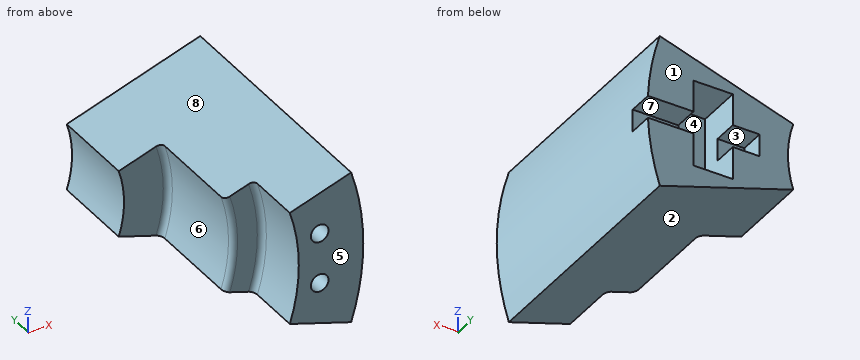
Autodesk Inventor part; units mm, degrees
ref_plane "YZ Plane" through (0, 0, 0) normal (1, 0, 0) x (0, 1, 0)
ref_plane "XZ Plane" through (0, 0, 0) normal (0, 1, 0) x (-1, 0, 0)
ref_plane "XY Plane" through (0, 0, 0) normal (0, 0, 1) x (1, 0, 0)
sketch "Эскиз3" plane through (0, 0, 0) normal (0, 0, 1) x (1, 0, 0)
  line L0 (28.4814, 0) -> (32, 0)
  line L1 (26.4814, 18.1962) -> (19.4814, 18.1962)
  line L2 (19.4814, 18.1962) -> (19.4814, 33.1962)
  line L3 (27.4814, 17.1962) -> (27.4814, 1)
  line L4 (33, -1) -> (33, -10.35)
  line L5 (33, -10.35) -> (44.4955, -10.35)
  line L6 (109.4355, -10.35) -> (-108.0344, -10.35)
  arc A0 (33, -1) -> (32, 0) centre (32, -1) ccw
  arc A1 (27.4814, 1) -> (28.4814, 0) centre (28.4814, 1) ccw
  arc A2 (27.4814, 17.1962) -> (26.4814, 18.1962) centre (26.4814, 17.1962) ccw
  line L7 (19.4814, 33.1962) -> (44.4955, 33.1962)
  line L8 (44.4955, 33.1962) -> (44.4955, -10.35)
  point P0 (27.4814, 18.1962)
  point P1 (27.4814, 0)
  dimension "d25" = 8
  dimension "d42" = 15
  dimension "d44" = 1
  dimension "d45" = 1
  dimension "d54" = 3.5186
  dimension "d55" = 25.0142
sketch "Эскиз4" plane through (0, 0, 0) normal (0, 1, 0) x (-1, 0, 0)
  arc A0 (-24.7386, 8) -> (-24.7386, -8) centre (0, 0) ccw
  dimension "d31" = 26
sweep "Сдвиг1" add profiles "Эскиз3" path "Эскиз4"
sketch "Эскиз8" plane through (0, -10.35, 0) normal (0, -1, 0) x (1, 0, 0)
  arc A0 (31.399, -10.1538) -> (31.399, 10.1538) centre (0, 0) ccw
  arc A1 (35.205, -11.3846) -> (35.205, 11.3846) centre (0, 0) ccw construction
  line L0 (42.3369, -13.6909) -> (31.399, -10.1538)
  circle A2 centre (36.723, -4.5186) radius 1.575
  circle A3 centre (36.723, 4.5186) radius 1.575
  line L1 (31.399, 10.1538) -> (42.3369, 13.6909)
  point P0 (0, 0)
  dimension "d46" = 4
  dimension "d47" = 3.15
  dimension "d48" = 3.15
  dimension "d49" = 7
  dimension "d50" = 7
extrude "Выдавливание4" cut sketch "Эскиз8" against normal blind 10
sketch "Эскиз9" plane through (0, 33.1962, 0) normal (0, 1, 0) x (1, 0, 0)
  point P0 (0, 0)
ref_plane "РабПлоскость1" through (0, -10.35, 0) normal (0, 0, 1) x (0, 1, 0)
sketch "Эскиз10" plane through (0, -10.35, 0) normal (0, 0, 1) x (0, 1, 0)
  line L0 (47.9462, -48.5362) -> (39.1462, -48.5362)
  line L1 (39.1462, -48.5362) -> (39.1462, -24.5362)
  line L2 (39.1462, -24.5362) -> (47.9462, -24.5362)
  line L3 (47.9462, -24.5362) -> (47.9462, -48.5362)
  line L4 (43.5462, -42.3369) -> (43.5462, -18.5362)
  line L5 (47.9462, -48.5362) -> (39.1462, -24.5362) construction
  line L6 (39.1462, -48.5362) -> (47.9462, -24.5362) construction
  line L7 (28.5462, -18.5362) -> (43.5462, -18.5362)
  point P0 (10.35, 0)
  point P1 (43.5462, -36.5362)
  dimension "d61" = 8.8
  dimension "d68" = 24
  dimension "d69" = 6
extrude "Выдавливание5" cut sketch "Эскиз10" along normal mid plane 4
sketch "Эскиз11" plane through (0, 33.1962, 0) normal (0, 1, 0) x (1, 0, 0)
  line L0 (34.8211, -6.1599) -> (30.8211, -6.1599)
  line L1 (30.8211, -6.1599) -> (30.8211, -0.8676)
  line L2 (30.8211, -0.8676) -> (34.8211, -0.8676)
  line L3 (34.8211, -0.8676) -> (34.8211, -6.1599)
  line L4 (30.8211, 6.3599) -> (34.8211, 6.3599)
  line L5 (34.8211, 6.3599) -> (34.8211, 1.0676)
  line L6 (34.8211, 1.0676) -> (30.8211, 1.0676)
  line L7 (30.8211, 1.0676) -> (30.8211, 6.3599)
  line L8 (36.3211, 7.8599) -> (29.3211, 7.8599)
  line L9 (29.3211, 7.8599) -> (29.3211, -0.4324)
  line L10 (29.3211, -0.4324) -> (36.3211, -0.4324)
  line L11 (36.3211, -0.4324) -> (36.3211, 7.8599)
  line L12 (36.3211, -7.6599) -> (29.3211, -7.6599)
  line L13 (29.3211, -7.6599) -> (29.3211, 0.6324)
  line L14 (29.3211, 0.6324) -> (36.3211, 0.6324)
  line L15 (36.3211, 0.6324) -> (36.3211, -7.6599)
  point P0 (0, 0)
  point P1 (29.3211, -0.4324)
  dimension "d66" = 1.5
  dimension "d67" = 1.5
extrude "Выдавливание6" cut sketch "Эскиз11" against normal blind 8 contours L0 L1 L2 L3 | L4 L5 L6 L7 | L11 L14 L9 L8 | L11 L10 L9 L14 | L15 L12 L13 L10
properties part number "креп_подш"
The model under review builds one solid part; all positions refer to its coordinate system, in mm. Face numbers are marked on the shaded views. A direction names the side the tool comes from. Give positions to 0.01 mm unless a question says otherwise; leave off trailing zeros. Loops run counter-clockwise (first coordinate to the right, second up) from the corner with the lowest first, then second, coordinate; pieces in that order, holes last. Notation, with made-up numbers: (7.5, 69) -> (56.5, 69) arc R21 ccw to (56.5, 82) -> close; hole circle Ø4 at (49.5, -16). An arc over 180 degrees is marked (long way). Answer as a JSON object with one key per item and string values. Group by question number.
Q1. Take a section at C-C (x = 39.5). Write out the cut boundary in (y, z), plus the area to 3 significant figures.
Q2. Take a section at D-D (y = -4). State how many separate pieces and enclosed holes the cut face has, plus the area to 3 significant figures.
Q3. Draft analysis for pull direction Z (two halves, no side actions). For the marked faces 1, 2 and 3, state which applies: pulls with the +Z half, pulls with the -Z half, needs draft (parallel to the pull), parting line crosses it, or undercut.
Q4. Take a section at A-A (y = 28). Write out the cut boundary in (x, z).
Q5. Tool access review of the marked faces 4, 5, 6, 7 and 8: name each direction out of +Z, -Z, +X, -X, +Y, -Y from which nothing blocks a thin tool from reaching the whole face with its end or side.
Q6. Insertion check: pin 1 (4.5 mm diameter, centred on x = 41, z = 0, fed in from +Y); pin 2 (2.5 mm diameter, centred on y = 30, z = 1.5, fed in from +X); pin 3 (5 mm diameter, centred on x = 27.5, y = 31.5, fed in from +Z); pin 4 (2.5 mm diameter, centred on x = 30, z = 4, fed in from -Y). Each pin has a flat end and moves straight along its axis. Give the tip position at first contact, or say it passes through.
Q7. Take a section at B-B (y = 2.5). Write out the cut boundary in (x, z).
Q8. Wall thickness on line 1 along Y through (x, z) = (33, -5); line 2 along Y through (x, z) = (21.75, -5); line 3 along Z through (x, y) = (34.75, 25): over which ranges is each line inside the solid? List them lowest first.
Answer below:
{
 "1": {"outline": "(-10.35, -12.77) -> (33.2, -12.77) -> (33.2, -2) -> (28.8, -2) -> (28.8, 2) -> (33.2, 2) -> (33.2, 12.77) -> (-10.35, 12.77) -> close", "area": "1,090 mm2"},
 "2": {"separate pieces": "1", "enclosed holes": "2", "area": "263 mm2"},
 "3": {"face 1": "needs draft", "face 2": "pulls with the -Z half", "face 3": "undercut"},
 "4": {"outline": "(18.54, -5.99) -> (42.34, -13.69) arc R44.5 ccw to (42.34, 13.69) -> (18.54, 5.99) arc R19.48 cw to start; hole (29.32, -7.86) -> (36.32, -7.86) -> (36.32, 7.66) -> (29.32, 7.66) -> close"},
 "5": {"face 4": "+Y", "face 5": "+Z, -Z, +X, -X, -Y", "face 6": "-X, -Y", "face 7": "+X, +Y", "face 8": "+Z, -X, +Y, -Y"},
 "6": {"pin 1": "stops at y = 33.2", "pin 2": "stops at x = 44.48", "pin 3": "stops at z = 9.7", "pin 4": "stops at y = 0"},
 "7": {"outline": "(26.15, -8.46) -> (42.34, -13.69) arc R44.5 ccw to (42.34, 13.69) -> (26.15, 8.46) arc R27.48 cw to start"},
 "8": {"line 1": "y = -10.35 to 25.2", "line 2": "y = 18.2 to 33.2", "line 3": "z = -11.24 to 11.24"}
}
